Geometry check sheet. Reference: the model listing, model coordinates, mm. A direction names the side the tool comes from. Round coordinates to 2 decimals unless told otherwise and drop trailing zeros. Write each loop counter-clockwise with the first axis right and the second up, starting at its lowest first coordinate (ties: lowest second). Pieces come first, ordered by that corner, then holes.
Item 1: Depth check by flat-ended pin: P1, Ø10, axis at x = -22, y = -14.5, coming from the +Z side; P2, Ø4, axis at y = 20.5, z = -11.5, coming from the -X side; P3, Ø3, axis at y = -20.5, z = -74.5, coming from the +X side; P4, Ø3.5, axis at x = -24.75, y = -24.75, coming from the -Z side. Enter the tip coordinate at first touch or a pass-through.
Item 2: Scan lines: probe 1 along Z at (x, y) = (-12, -18); probe 2 along Z at (x, y) = (22, -18.5); probe 3 along Y at (x, z) = (-20.5, -31). Record each from-to range of solid material in increasing order.
Item 3: Cross-section at C-C (z = -75). Enter the section's corners in (x, y).
Item 4: Access from +Z, -Z, +X, -X, +Y, -Y to the whole of each face (thin tool, end or side, straight path). Record for faces 1 (the face through (-23, -23, 0)), 2 (the face through (-23, 22, 0)), 3 (the face through (-13.797, -26.526, -105.056)).
Item 5: Cross-section at B-B (y = -5.5). Enter the section's corners in (x, z), then the cut area to 3 significant figures.
Item 6: Draft check along X on faces 4 (the face through (0, 30, 3)), 5 (the face through (0, -4, 18)), 6 (the face through (-23.539, -26.646, 2.958)). Enter one of: pulls with the +X half, pulls with the -X half, needs draft (parallel to the pull), parting line crosses it, or undercut.
Item 7: Cross-section at A-A (x = 19). Enter the section's corners in (y, z), then the cut area to 3 significant figures.
Autodesk Inventor part; units mm, degrees
ref_plane "YZ Plane" through (0, 0, 0) normal (1, 0, 0) x (0, 1, 0)
ref_plane "XZ Plane" through (0, 0, 0) normal (0, 1, 0) x (-1, 0, 0)
ref_plane "XY Plane" through (0, 0, 0) normal (0, 0, 1) x (1, 0, 0)
sketch "스케치1" plane through (0, 0, 0) normal (0, 0, 1) x (1, 0, 0)
  line L0 (-30, -30) -> (30, -30)
  line L1 (30, -30) -> (30, 30)
  line L2 (30, 30) -> (-30, 30)
  line L3 (-30, 30) -> (-30, -30)
  line L4 (-30, -30) -> (30, 30) construction
  line L5 (30, -30) -> (-30, 30) construction
  circle A0 centre (0, 0) radius 30
  circle A1 centre (-24.7487, 24.7487) radius 2.25
  circle A2 centre (0, 0) radius 35 construction
  circle A3 centre (-24.7487, -24.7487) radius 2.25
  circle A4 centre (24.7487, -24.7487) radius 2.25
  circle A5 centre (24.7487, 24.7487) radius 2.25
  dimension "d3" = 70
  dimension "d0" = 60
  dimension "d1" = 60
  dimension "d2" = 4.5
  dimension "d6" = 360
extrude "돌출1" add sketch "스케치1" along normal blind 6
extrude "돌출2" add sketch "스케치1" against normal blind 109 contours A0
sketch "스케치2" plane through (0, 0, -109) normal (0, 0, -1) x (-1, 0, 0)
  circle A0 centre (0, 0) radius 30
  circle A1 centre (0, 0) radius 29.9
  dimension "d12" = 0.1
extrude "돌출3" cut sketch "스케치2" against normal blind 8
sketch "스케치3" plane through (0, 0, 6) normal (0, 0, 1) x (1, 0, 0)
  circle A0 centre (0, 0) radius 27
  dimension "d15" = 54
extrude "돌출4" add sketch "스케치3" along normal blind 2
sketch "스케치4" plane through (0, 0, 8) normal (0, 0, 1) x (1, 0, 0)
  circle A0 centre (0, 0) radius 4
  line L0 (-2.6458, 3) -> (2.6458, 3)
  line L1 (0, 3) -> (0, -4)
  dimension "d18" = 8
  dimension "d19" = 7
extrude "돌출5" add sketch "스케치4" along normal blind 20 contours A0 L1 L0 | A0 L0 L1
extrude "돌출6" add sketch "스케치4" along normal blind 5 contours L0 A0
fillet "모깎기1" radius 5 4 edges at (-30, 30, 3) (30, 30, 3) (-30, -30, 3) (30, -30, 3)
properties part number "중형 모터 MB60080-2430 DC24V"
Resolved:
1. P1: stops at z = 8
1. P2: stops at x = -23.62
1. P3: stops at x = 23.22
1. P4: passes through
2. probe 1: z = -109 to 8
2. probe 2: z = -109 to 6
2. probe 3: y = -21.9 to 21.9
3. outline: circle Ø60 at (0, 0)
4. face 1: -Z, -X, -Y
4. face 2: -Z, -X, +Y
4. face 3: -Z
5. outline: (-30, 0) - (-29.49, 0) - (-29.49, -101) - (-29.39, -101) - (-29.39, -109) - (29.39, -109) - (29.39, -101) - (29.49, -101) - (29.49, 0) - (30, 0) - (30, 6) - (26.43, 6) - (26.43, 8) - (-26.43, 8) - (-26.43, 6) - (-30, 6) - close
5. area: 6,890 mm2
6. face 4: needs draft
6. face 5: parting line crosses it
6. face 6: undercut
7. outline: (-30, 0) - (-23.22, 0) - (-23.22, -101) - (-23.09, -101) - (-23.09, -109) - (23.09, -109) - (23.09, -101) - (23.22, -101) - (23.22, 0) - (30, 0) - (30, 6) - (19.18, 6) - (19.18, 8) - (-19.18, 8) - (-19.18, 6) - (-30, 6) - close
7. area: 5,500 mm2
